from build123d import *

# Parameters (mm, degrees)
Y_KSEKLIK_EKSTR_ZYON1_DEPTH = 150


with BuildPart() as part:
    # Çizim1 → Yükseklik-Ekstrüzyon1 (new body)
    with BuildSketch(Plane.XY):
        with BuildLine():
            ThreePointArc((-1.077539734, -38.836840411), (10.094920531, -17.484915258), (34.172460266, -18.485243422))
            ThreePointArc((34.172460266, -18.485243422), (69.5, 0), (34.172460266, 18.485243422))
            ThreePointArc((34.172460266, 18.485243422), (10.094920531, 17.484915258), (-1.077539734, 38.836840411))
            ThreePointArc((-1.077539734, 38.836840411), (-34.75, 60.188765563), (-33.094920531, 20.351596989))
            ThreePointArc((-33.094920531, 20.351596989), (-20.189841062, 0), (-33.094920531, -20.351596989))
            ThreePointArc((-33.094920531, -20.351596989), (-34.75, -60.188765563), (-1.077539734, -38.836840411))
        make_face()
        with BuildLine():
            ThreePointArc((-5.558451419, 10.635018469), (-3.708203932, 11.412678196), (-1.754225354, 11.871086446))
            Line((-1.754225354, 11.871086446), (-1.1256228, 9.936446715))
            ThreePointArc((-1.1256228, 9.936446715), (3.090169944, 9.510565163), (6.751144813, 7.377129775))
            Line((6.751144813, 7.377129775), (8.396847665, 8.572802885))
            ThreePointArc((8.396847665, 8.572802885), (9.708203932, 7.053423028), (10.747988674, 5.336734907))
            Line((10.747988674, 5.336734907), (9.102285822, 4.141061797))
            ThreePointArc((9.102285822, 4.141061797), (9.77299489, 2.118624763), (10, 0))
            ThreePointArc((10, 0), (9.77299489, -2.118624763), (9.102285822, -4.141061797))
            Line((9.102285822, -4.141061797), (10.747988674, -5.336734907))
            ThreePointArc((10.747988674, -5.336734907), (9.708203932, -7.053423028), (8.396847665, -8.572802885))
            Line((8.396847665, -8.572802885), (6.751144813, -7.377129775))
            ThreePointArc((6.751144813, -7.377129775), (3.090169944, -9.510565163), (-1.1256228, -9.936446715))
            Line((-1.1256228, -9.936446715), (-1.754225354, -11.871086446))
            ThreePointArc((-1.754225354, -11.871086446), (-3.708203932, -11.412678196), (-5.558451419, -10.635018469))
            Line((-5.558451419, -10.635018469), (-4.929848865, -8.700378737))
            ThreePointArc((-4.929848865, -8.700378737), (-8.090169944, -5.877852523), (-9.797958971, -2))
            Line((-9.797958971, -2), (-11.832159566, -2))
            ThreePointArc((-11.832159566, -2), (-12, 0), (-11.832159566, 2))
            Line((-11.832159566, 2), (-9.797958971, 2))
            ThreePointArc((-9.797958971, 2), (-8.090169944, 5.877852523), (-4.929848865, 8.700378737))
            Line((-4.929848865, 8.700378737), (-5.558451419, 10.635018469))
        make_face(mode=Mode.SUBTRACT)
    extrude(amount=-Y_KSEKLIK_EKSTR_ZYON1_DEPTH)


solid = part.part
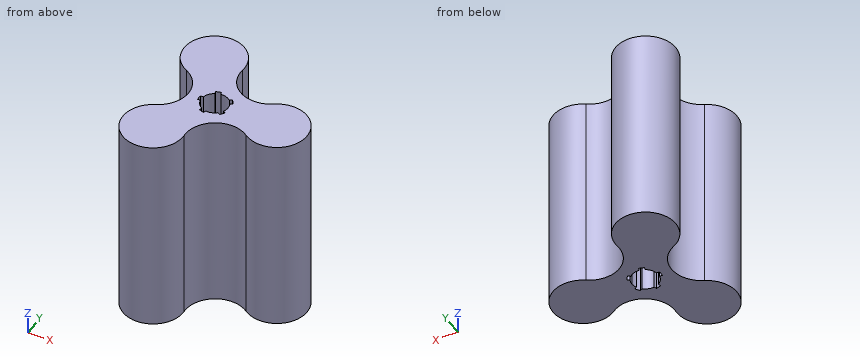
Model file for the job. Use its own axes, mm. Give positions to 0.01 mm unless a question says otherwise; leave off trailing zeros. Order: outer loops, then holes, each group sorted by start corner. A loop starts at its lowest first (then second) coordinate and runs counter-clockwise, first axis right, second up. Notation, with made-up numbers: (-39.75, 37) - (-33.75, 37) arc R27 ccw to (-33.75, 76) - close; hole circle Ø6 at (-26.75, -5.75). An arc over 180 degrees is marked (long way). Return JSON: item names as keys, results as strings.
1) Cut at A-A, the plane x = -23.5. Give the cut face in (y, z), plus the area to 3 significant figures.
Geometry says:
{"outline": "(-63.2, -150) - (-11.75, -150) - (-11.75, 0) - (-63.2, 0) - close; (11.75, -150) - (63.2, -150) - (63.2, 0) - (11.75, 0) - close", "area": "15,400 mm²"}
2) Probe line 1 (Y direction, x = -25.5, z = -134.5); line 2 (X direction, y = 40.5, z = -135); line 3 (X direction, y = -7, z = -75). List the from-to ranges inside material, lowest first. Write a range as from..to.
Geometry says:
{"line 1": "-63.11..-14.52, 14.52..63.11", "line 2": "-46..-1", "line 3": "-21.31..-7.14, 9.75..68.38"}
3) Flat gauge pins, fed straight in: P1, Ø1.5, axis at y = -9.5, z = -111.5, coming from the -X side; P2, Ø8, axis at x = 46, z = -35.5, coming from the -Y side; P3, Ø2, axis at y = -15, z = -125.5, coming from the -X side. Where does each tip first touch, or does it go through?
Geometry says:
{"P1": "x = -22.66", "P2": "y = -22.5", "P3": "x = -26.87"}
4) Cut at D-D, the plane y = 47.5. Give the cut face in (x, z).
Geometry says:
{"outline": "(-44.95, -150) - (-2.05, -150) - (-2.05, 0) - (-44.95, 0) - close"}
5) Cut at B-B, the plane z = -48. Give the cut face in (x, y).
Geometry says:
{"outline": "(-33.09, -20.35) arc R22.5 ccw (long way) to (-1.08, -38.84) arc R22.5 cw to (34.17, -18.49) arc R22.5 ccw (long way) to (34.17, 18.49) arc R22.5 cw to (-1.08, 38.84) arc R22.5 ccw (long way) to (-33.09, 20.35) arc R22.5 cw to start; hole (-11.83, -2) - (-9.8, -2) arc R10 ccw to (-4.93, -8.7) - (-5.56, -10.64) arc R12 ccw to (-1.75, -11.87) - (-1.13, -9.94) arc R10 ccw to (6.75, -7.38) - (8.4, -8.57) arc R12 ccw to (10.75, -5.34) - (9.1, -4.14) arc R10 ccw to (9.1, 4.14) - (10.75, 5.34) arc R12 ccw to (8.4, 8.57) - (6.75, 7.38) arc R10 ccw to (-1.13, 9.94) - (-1.75, 11.87) arc R12 ccw to (-5.56, 10.64) - (-4.93, 8.7) arc R10 ccw to (-9.8, 2) - (-11.83, 2) arc R12 ccw to start"}
6) Cut at C-C, the plane x = -37.5. Give the cut face in (y, z), plus the area to 3 significant figures.
Geometry says:
{"outline": "(-58.32, -150) - (-23.09, -150) - (-23.09, 0) - (-58.32, 0) - close; (23.09, -150) - (58.32, -150) - (58.32, 0) - (23.09, 0) - close", "area": "10,600 mm²"}
